```python
from build123d import *

# Parameters (mm, degrees)
SKETCH1_W           = 122
SKETCH1_H           = 77
BOSS_EXTRUDE1_DEPTH = 9
SKETCH2_W           = 109
SKETCH2_H           = 66
CUT_EXTRUDE1_DEPTH  = 1
BOSS_EXTRUDE2_DEPTH = 2
SKETCH4_R           = 1.75
CUT_EXTRUDE3_DEPTH  = 4
SKETCH5_W           = 12
SKETCH5_H           = 4
SKETCH5_W_2         = 20
SKETCH5_H_2         = 5
CUT_EXTRUDE4_DEPTH  = 2
SKETCH11_W          = 12
SKETCH11_H          = 4
BOSS_EXTRUDE4_DEPTH = 10
SKETCH12_W          = 2.415928069
SKETCH12_H          = 12
BOSS_EXTRUDE5_DEPTH = 4.5
SKETCH13_W          = 12
SKETCH13_H          = 2.350282926
BOSS_EXTRUDE6_DEPTH = 14
SKETCH11_2_W        = 12
SKETCH11_2_H        = 4
BOSS_EXTRUDE7_DEPTH = 14


with BuildPart() as part:
    # Sketch1 → Boss-Extrude1 (new body)
    with BuildSketch(Plane(origin=(0, 0, 0), x_dir=(1, 0, 0), z_dir=(0, 1, 0))):
        with Locations((61, 38.5)):
            Rectangle(SKETCH1_W, SKETCH1_H)
    extrude(amount=BOSS_EXTRUDE1_DEPTH)

    # Sketch2 → Cut-Extrude1 (cut)
    with BuildSketch(Plane(origin=(0, 9, 0), x_dir=(1, 0, 0), z_dir=(0, 1, 0))):
        with Locations((61, 38.5)):
            Rectangle(SKETCH2_W, SKETCH2_H)
    extrude(amount=-CUT_EXTRUDE1_DEPTH, mode=Mode.SUBTRACT)

    # Sketch3 → Boss-Extrude2 (add)
    with BuildSketch(Plane.XZ):
        with BuildLine():
            Line((0, -81.66), (0, -72.34))
            ThreePointArc((0, -72.34), (4, -68.34), (8, -72.34))
            Line((8, -72.34), (8, -81.66))
            ThreePointArc((8, -81.66), (4, -85.66), (0, -81.66))
        make_face()
        with BuildLine():
            Line((122, -81.66), (122, -72.34))
            ThreePointArc((122, -72.34), (118, -68.34), (114, -72.34))
            Line((114, -72.34), (114, -81.66))
            ThreePointArc((114, -81.66), (118, -85.66), (122, -81.66))
        make_face()
        with BuildLine():
            Line((0, 4.66), (0, -4.66))
            ThreePointArc((0, -4.66), (4, -8.66), (8, -4.66))
            Line((8, -4.66), (8, 4.66))
            ThreePointArc((8, 4.66), (4, 8.66), (0, 4.66))
        make_face()
        with BuildLine():
            Line((122, 4.66), (122, -4.66))
            ThreePointArc((122, -4.66), (118, -8.66), (114, -4.66))
            Line((114, -4.66), (114, 4.66))
            ThreePointArc((114, 4.66), (118, 8.66), (122, 4.66))
        make_face()
    extrude(amount=-BOSS_EXTRUDE2_DEPTH)

    # Sketch4 → Cut-Extrude3 (cut)
    with BuildSketch(Plane.XZ):
        with Locations(Location((4, -81.66, 0), (0, 0, 270))):
            Circle(SKETCH4_R)
        with Locations(Location((118, -81.66, 0), (0, 0, 90))):
            Circle(SKETCH4_R)
        with Locations(Location((4, 4.66, 0), (0, 0, 90))):
            Circle(SKETCH4_R)
        with Locations(Location((118, 4.66, 0), (0, 0, 270))):
            Circle(SKETCH4_R)
    extrude(amount=-CUT_EXTRUDE3_DEPTH, mode=Mode.SUBTRACT)

    # Sketch5 → Cut-Extrude4 (cut)
    with BuildSketch(Plane(origin=(122, 0, 0), x_dir=(0, 0, -1), z_dir=(1, 0, 0))):
        with Locations((67.5, 2.5)):
            Rectangle(SKETCH5_W, SKETCH5_H)
        with Locations((47, 4.5)):
            Rectangle(SKETCH5_W_2, SKETCH5_H_2)
    extrude(amount=-CUT_EXTRUDE4_DEPTH, mode=Mode.SUBTRACT)



with BuildPart() as body_2:
    # Sketch11 → Boss-Extrude4 (new body)
    with BuildSketch(Plane(origin=(122, 0, 0), x_dir=(0, 0, -1), z_dir=(1, 0, 0))):
        with Locations((67.5, 2.5)):
            Rectangle(SKETCH11_W, SKETCH11_H)
    extrude(amount=BOSS_EXTRUDE4_DEPTH)

    # Sketch12 → Boss-Extrude5 (add)
    with BuildSketch(Plane.XZ.offset(-0.5)):
        with Locations((130.792035966, -67.5)):
            Rectangle(SKETCH12_W, SKETCH12_H)
    extrude(amount=BOSS_EXTRUDE5_DEPTH)

    # Sketch13 → Boss-Extrude6 (add)
    with BuildSketch(Plane.ZY.offset(-129.584071931)):
        with Locations((-67.5, -2.824858537)):
            Rectangle(SKETCH13_W, SKETCH13_H)
    extrude(amount=BOSS_EXTRUDE6_DEPTH)


with BuildPart() as part_1:
    add(part.part)

    add(body_2.part)  # Boss-Extrude7 merges body 2
    # Sketch11_2 → Boss-Extrude7 (add)
    with BuildSketch(Plane(origin=(122, 0, 0), x_dir=(0, 0, -1), z_dir=(1, 0, 0))):
        with Locations((67.5, 2.5)):
            Rectangle(SKETCH11_2_W, SKETCH11_2_H)
    extrude(amount=-BOSS_EXTRUDE7_DEPTH)


solid = part_1.part
```
Could you check a few things on this model? Use its own coordinates, in mm. A direction names the side the tool comes from. Round coordinates to 2 decimals unless told otherwise and drop trailing zeros. Loops run counter-clockwise (first coordinate to the right, second up) from the corner with the lowest first, then second, coordinate; pieces in that order, holes last. Notation, with made-up numbers: M -23,37.5 L 30,37.5 A35 cw 30,71.5 Z; hole C 88.5,10 d4. An arc over 180 degrees is marked long. Write item = value, one per line.
1. Will these pins go through, and if not, where does the flat tip stop? P1, Ø4.5, axis at x = 51.5, y = 4, coming from the +Z side; P2, Ø1.6, axis at y = 1.5, z = -80.5, coming from the +X side; P3, Ø1.2, axis at y = -3, z = -69, coming from the -X side.
Results below:
P1 = 0
P2 = 122
P3 = 115.58
2. Which directions (+Z, -Z, +X, -X, +Y, -Y) give clear straight access to the entire face, cutting with the end or side of a thin tool? Please do faces 1 (the face through (126, 1, -61.5)), 2 (the face through (126, 0.5, -67)), 3 (the face through (127, 4.5, -67)), 4 (the face through (126, 1, -73.5)), 5 (the face through (118, 2, 2)).
Results below:
face_1 = +Z, +X, -Y
face_2 = +Z, -Z
face_3 = +Z, -Z, +X, +Y
face_4 = -Z, +X, -Y
face_5 = +Z, +X, -X, +Y
3. I want a section at D-D, the plane z = -38.5. Write out the boundary of the cut face in (x, y).
Results below:
outline = M 0,0 L 122,0 L 122,2 L 120,2 L 120,7 L 122,7 L 122,9 L 115.5,9 L 115.5,8 L 6.5,8 L 6.5,9 L 0,9 Z
4. Thinking about a two-plate mould opening in Z: for faces 6 (the face through (123, -1.65, -68)), 7 (the face through (60, 8, -39)), 8 (the face through (117.91, 0.99, 8.66)), which applies, +Z half, -Z half, draft (parallel to the pull), parting line (faces both ways), or undercut?
Results below:
face_6 = draft
face_7 = undercut
face_8 = +Z half
5. I need wall thicknesses on probe 1 along Z at (x, y) = (118, 1.3); probe 2 along X at (y, z) = (0.7, 4.66); probe 3 along X at (y, z) = (0.5, -81). Which ranges of each line are inside material? Lowest first, please.
Results below:
probe_1 = -85.66 to -83.41, -79.91 to 2.91, 6.41 to 8.66
probe_2 = 0 to 2.25, 5.75 to 8, 114 to 116.25, 119.75 to 122
probe_3 = 0 to 2.38, 5.62 to 8, 114 to 116.38, 119.62 to 122
6. I want a section at A-A, the plane x = 118. Write out the boundary of the cut face in (y, z).
Results below:
outline = M -4,-73.5 L -1.65,-73.5 L -1.65,-61.5 L -4,-61.5 Z; M 0,-85.66 L 2,-85.66 L 2,-83.41 L 0,-83.41 Z; M 0,-79.91 L 2,-79.91 L 2,-77 L 9,-77 L 9,0 L 2,0 L 2,2.91 L 0,2.91 Z; M 0,6.41 L 2,6.41 L 2,8.66 L 0,8.66 Z
7. I want a section at B-B, the plane z = -26. Write out the boundary of the cut face in (x, y), and give its area (3 significant figures).
Results below:
outline = M 0,0 L 122,0 L 122,9 L 115.5,9 L 115.5,8 L 6.5,8 L 6.5,9 L 0,9 Z
area = 989 mm²
8. I want a section at C-C, the plane x = 96. Write out the boundary of the cut face in (y, z).
Results below:
outline = M 0,-77 L 9,-77 L 9,-71.5 L 8,-71.5 L 8,-5.5 L 9,-5.5 L 9,0 L 0,0 Z
